Input: part model. Units: mm. Frame: model coordinates. Face numbers are marked on the shaded views. A direction names the side the tool comes from. Round coordinates to 2 decimals unless told otherwise and drop trailing zeros. Loops run counter-clockwise (first coordinate to the right, second up) from the corner with the lowest first, then second, coordinate; pieces in that order, holes last.
(1) Cut plane C-C, the plane y = 3.75. Output: boundary loops of the cut face in (x, z).
(2) First-contact query: pin 1 Ø4 at (x, z) = (1.5, 3) entering from -Y; pin 2 Ø1.6 at (y, z) = (-9.5, 2.5) entering from -X; pin 3 Ø1 at (x, y) = (-3.5, 4) entering from -Z; pin 4 Ø1.1 at (y, z) = (-9, 2) entering from +X. Flat tips, straight axial feed; report the tip coordinate or a pass-through.
(3) Cut plane D-D, the plane z = 4.25. Output: boundary loops of the cut face in (x, y), and give its area (3 significant figures).
(4) Draft query along X for the marked faces 1, 2 and 3. Return one class per face: released by +X, released by -X, zero draft, split by the parting line, or undercut.
(5) Cut plane A-A, the plane x = 0. Output: boundary loops of the cut face in (y, z), and give its area (3 significant figures).
(6) Cut plane B-B, the plane z = 0. Output: boundary loops of the cut face in (x, y).
(7) Line query: line 1 (X direction, y = 5.95, z = 0); line 2 (X direction, y = 2.5, z = -4.25); line 3 (Z direction, x = 0, y = 7.3). Output: solid intervals per line, ascending.
(8) Access query for the marked faces 4 and 5. Directions: +Z, -Z, +X, -X, +Y, -Y. A direction counts if a zero-diameter tool reaches every point of the face in a straight line with its end or side. Return the directions, or none.
Autodesk Inventor part; units mm, degrees
ref_plane "YZ Plane" through (0, 0, 0) normal (1, 0, 0) x (0, 1, 0)
ref_plane "XZ Plane" through (0, 0, 0) normal (0, 1, 0) x (-1, 0, 0)
ref_plane "XY Plane" through (0, 0, 0) normal (0, 0, 1) x (1, 0, 0)
sketch "スケッチ1" plane through (0, 0, 0) normal (0, 0, 1) x (1, 0, 0)
  line L0 (-14, 8.973) -> (14, 8.973)
  line L1 (14, 8.973) -> (14, -10.027)
  line L2 (4, -8.027) -> (9, -0.027)
  line L3 (-9, -0.027) -> (-4, -8.027)
  line L4 (-14, -10.027) -> (-14, 8.973)
  line L5 (-4, -8.027) -> (-4, -10.027)
  line L6 (-4, -10.027) -> (-14, -10.027)
  line L7 (4, -8.027) -> (4, -10.027)
  line L8 (4, -10.027) -> (14, -10.027)
  line L9 (0, -13.827) -> (0, 12.773)
  line L10 (-9, -0.027) -> (-9, 4.973)
  line L11 (-9, 4.973) -> (9, 4.973)
  line L12 (9, 4.973) -> (9, -0.027)
  point P0 (0, 0)
  dimension "d1" = 8
  dimension "d2" = 18
  dimension "d3" = 10
  dimension "d6" = 2
  dimension "d7" = 5
  dimension "d8" = 4
  dimension "d9" = 15
extrude "押し出し1" add sketch "スケッチ1" along normal mid plane 12
sketch "スケッチ2" plane through (-14, 8.973, 6) normal (0, 1, 0) x (1, 0, 0)
  circle A0 centre (14, 6) radius 1.5
  dimension "d12" = 3
extrude "押し出し2" cut sketch "スケッチ2" against normal through all
fillet "フィレット1" radius 2 2 edges at (-4, -8.027, 0) (4, -8.027, 0)
chamfer "面取り1" distance 5 angle 45 2 edges at (-14, -10.027, 0) (14, -10.027, 0)
properties part number "gripper"
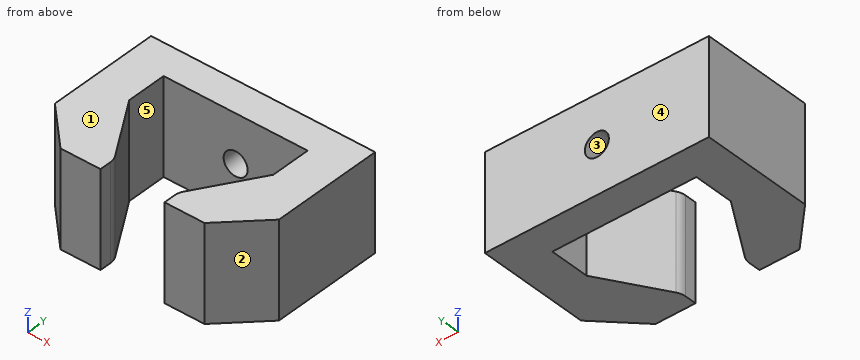
Reported:
1. outline: (-14, -6) - (-9, -6) - (-9, 6) - (-14, 6) - close; (9, -6) - (14, -6) - (14, 6) - (9, 6) - close
2. pin 1: stops at y = 4.97
2. pin 2: stops at x = -10.33
2. pin 3: passes through
2. pin 4: stops at x = 10.58
3. outline: (-14, -5.03) - (-9, -10.03) - (-4, -10.03) - (-4, -8.6) arc R2 ccw to (-4.3, -7.54) - (-9, -0.03) - (-9, 4.97) - (9, 4.97) - (9, -0.03) - (4.3, -7.54) arc R2 ccw to (4, -8.6) - (4, -10.03) - (9, -10.03) - (14, -5.03) - (14, 8.97) - (-14, 8.97) - close
3. area: 297 mm2
4. face 1: zero draft
4. face 2: released by +X
4. face 3: undercut
5. outline: (4.97, -6) - (8.97, -6) - (8.97, -1.5) - (4.97, -1.5) - close; (4.97, 1.5) - (8.97, 1.5) - (8.97, 6) - (4.97, 6) - close
5. area: 36.0 mm2
6. outline: (-14, -5.03) - (-9, -10.03) - (-4, -10.03) - (-4, -8.6) arc R2 ccw to (-4.3, -7.54) - (-9, -0.03) - (-9, 4.97) - (-1.5, 4.97) - (-1.5, 8.97) - (-14, 8.97) - close; (1.5, 4.97) - (9, 4.97) - (9, -0.03) - (4.3, -7.54) arc R2 ccw to (4, -8.6) - (4, -10.03) - (9, -10.03) - (14, -5.03) - (14, 8.97) - (1.5, 8.97) - close
7. line 1: x = -14 to -1.5, 1.5 to 14
7. line 2: x = -14 to -9, 9 to 14
7. line 3: z = -6 to -1.5, 1.5 to 6
8. face 4: +Z, -Z, +X, -X, +Y
8. face 5: +Z, -Z
